The figure shows three views and two pictorial views of one solid part (mm, origin at its lowest corner). Answer the questions. Coordinates: 2 decimals unless noted, no trailing zeros. Loops run counter-clockwise (first coordinate to the right, second up) from the corner with the lowest first, then second, coordinate; pieces in that order, holes last. Notation, with made-up numbers: M 88,35 L 146,35 A18 ccw 146,57 Z; hole C 62,72.25 d6. An arc over 180 degrees is marked long. Return JSON: item names as keys, results as strings. Group by question number.
1. The mould has two halves that part along X. Classify the marked faces 1 and 2: pulls with the +X half, pulls with the -X half, needs draft (parallel to the pull), parting line crosses it, or undercut.
2. Given P1, Ø5, axis at x = 4.35, y = 12.5, coming from the -Z side, flat-ended and moving along its own axis, determine where the tip first touches the part or whether it passes through.
3. Section A-A (x = 12.5) is taken. Write down the section's boundary in (y, z).
4. Section D-D (z = 0.4) is taken. Write down the section's boundary in (x, y), then the cut area to 3 significant figures.
5. Section C-C (z = 2.2) is taken. Count the separate pieces of the cut face and the enclosed holes in it, then the cut area to 3 significant figures.
6. Straight lines are drawn through the part: L1, parallel to Y at x = 12.5, z = 0.2; L2, parallel to Z at x = 21.25, y = 4; L3, parallel to Y at x = 10.75, z = 0.9. For each, find the intervals that lie inside material, in ascending order. Write a range as from..to.
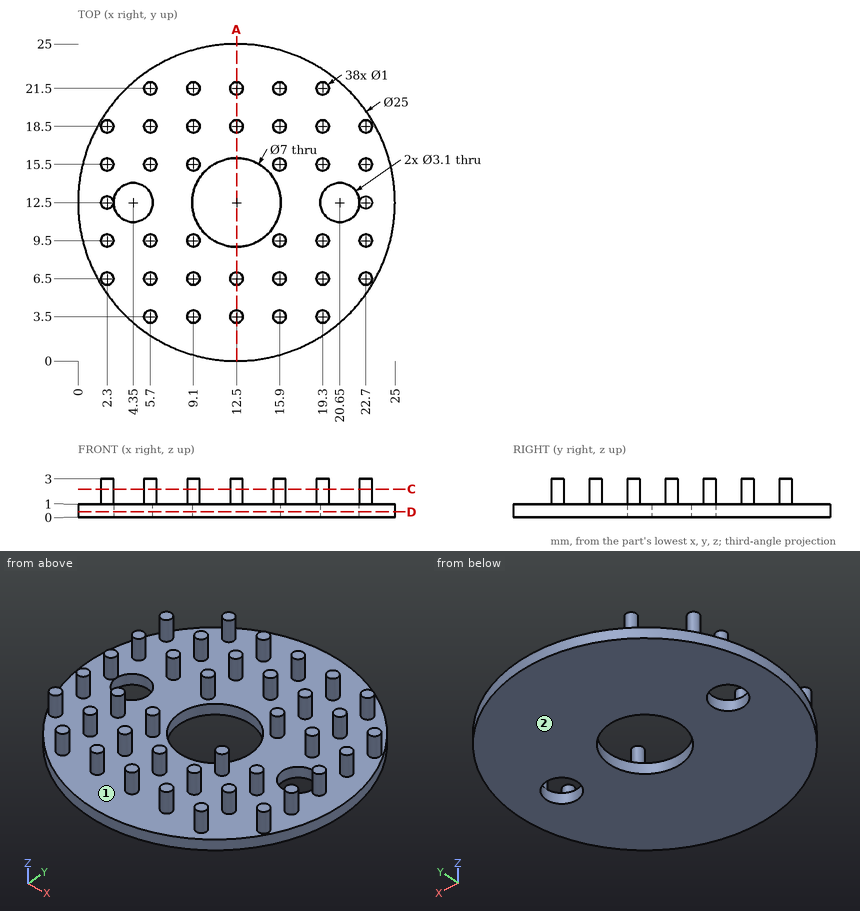
Worked out:
{
 "1": {"face 1": "undercut", "face 2": "needs draft"},
 "2": {"P1": "z = 0"},
 "3": {"outline": "M 0,0 L 9,0 L 9,1 L 7,1 L 7,3 L 6,3 L 6,1 L 4,1 L 4,3 L 3,3 L 3,1 L 0,1 Z; M 16,0 L 25,0 L 25,1 L 22,1 L 22,3 L 21,3 L 21,1 L 19,1 L 19,3 L 18,3 L 18,1 L 16,1 Z"},
 "4": {"outline": "C 12.5,12.5 d25; hole C 4.35,12.5 d3.1; hole C 12.5,12.5 d7; hole C 20.65,12.5 d3.1", "area": "437 mm^2"},
 "5": {"separate pieces": "38", "enclosed holes": "0", "area": "29.8 mm^2"},
 "6": {"L1": "0..9, 16..25", "L2": "0..1", "L3": "0.12..9.47, 15.53..24.88"}
}
